Verification items for the finished model (mm, model axes). Coordinates: 2 decimals unless noted, no trailing zeros. Order: outer loops, then holes, each group sorted by start corner. A loop starts at its lowest first (then second) coordinate and runs counter-clockwise, first axis right, second up. Notation, with made-up numbers: M 27.5,-29.75 L 56.5,-29.75 A16 ccw 56.5,-21.75 Z; hole C 85,12.5 d6. An arc over 180 degrees is marked long. Return JSON: item names as keys, results as strings. Group by question number.
1. Material ranges on line 1 along X through (y, z) = (0.95, 76.2); line 2 along Z through (x, y) = (-88.9, 1); line 3 along Z through (x, y) = (9, 0.3), recorded low to high.
2. Section check A-A, the plane z = -36.5. Record the cut outline in (x, y).
3. Section check B-B, the plane x = -46.5. Record the cut outline in (y, z).
4. Gauge pin test, flat end, axial feed: pin 1 (1.8 mm diameter, centred on x = -88.9, z = 76.2, fed in from -Y). Record the tip position at first contact, or that the pin passes through.
5. Section check C-C, the plane y = 0.4. Give the number of separate pieces and of enclosed holes in the cut face, plus the area to 3 significant figures.
```python
from build123d import *

# Parameters (mm, degrees)
SKETCH1_W           = 203.2
SKETCH1_H           = 172.72
BOSS_EXTRUDE1_DEPTH = 1.5875
CUT_EXTRUDE1_DEPTH  = 1.5875
SKETCH3_R           = 1.5
CUT_EXTRUDE2_DEPTH  = 1.5875
FILLET1_R           = 10


with BuildPart() as part:
    # Sketch1 → Boss-Extrude1 (new body)
    with BuildSketch(Plane(origin=(0, 0, 0), x_dir=(1, 0, 0), z_dir=(0, 1, 0))):
        Rectangle(SKETCH1_W, SKETCH1_H)
    extrude(amount=BOSS_EXTRUDE1_DEPTH)

    # Sketch2 → Cut-Extrude1 (cut)
    with BuildSketch(Plane(origin=(0, 1.5875, 0), x_dir=(1, 0, 0), z_dir=(0, 1, 0))):
        with BuildLine():
            Line((-56.337811401, 60.96), (56.337811401, 60.96))
            ThreePointArc((56.337811401, 60.96), (61.186538483, 57.180592348), (58.70513907, 51.555938272))
            Line((58.70513907, 51.555938272), (14.203966015, 27.635097742))
            ThreePointArc((14.203966015, 27.635097742), (0, 24.059468112), (-14.203966015, 27.635097742))
            Line((-14.203966015, 27.635097742), (-58.70513907, 51.555938272))
            ThreePointArc((-58.70513907, 51.555938272), (-61.186538483, 57.180592348), (-56.337811401, 60.96))
        make_face()
        with BuildLine():
            Line((-56.337811401, -60.96), (56.337811401, -60.96))
            ThreePointArc((56.337811401, -60.96), (61.186538483, -57.180592348), (58.70513907, -51.555938272))
            Line((58.70513907, -51.555938272), (14.203966015, -27.635097742))
            ThreePointArc((14.203966015, -27.635097742), (0, -24.059468112), (-14.203966015, -27.635097742))
            Line((-14.203966015, -27.635097742), (-58.70513907, -51.555938272))
            ThreePointArc((-58.70513907, -51.555938272), (-61.186538483, -57.180592348), (-56.337811401, -60.96))
        make_face()
        with BuildLine():
            Line((-68.832672331, 20.873835416), (-41.470344365, 6.16568642))
            ThreePointArc((-41.470344365, 6.16568642), (-37.784603101, 0), (-41.470344365, -6.16568642))
            Line((-41.470344365, -6.16568642), (-68.832672331, -20.873835416))
            ThreePointArc((-68.832672331, -20.873835416), (-73.765478674, -20.761430614), (-76.2, -16.469773687))
            Line((-76.2, -16.469773687), (-76.2, 16.469773687))
            ThreePointArc((-76.2, 16.469773687), (-73.765478674, 20.761430614), (-68.832672331, 20.873835416))
        make_face()
        with BuildLine():
            Line((41.470344365, 6.16568642), (68.832672331, 20.873835416))
            ThreePointArc((68.832672331, 20.873835416), (73.765478674, 20.761430614), (76.2, 16.469773687))
            Line((76.2, 16.469773687), (76.2, -16.469773687))
            ThreePointArc((76.2, -16.469773687), (73.765478674, -20.761430614), (68.832672331, -20.873835416))
            Line((68.832672331, -20.873835416), (41.470344365, -6.16568642))
            ThreePointArc((41.470344365, -6.16568642), (37.784603101, 0), (41.470344365, 6.16568642))
        make_face()
    extrude(amount=-CUT_EXTRUDE1_DEPTH, mode=Mode.SUBTRACT)

    # Sketch3 → Cut-Extrude2 (cut)
    with BuildSketch(Plane(origin=(0, 1.5875, 0), x_dir=(1, 0, 0), z_dir=(0, 1, 0))):
        with Locations(Location((-88.9, 76.2, 0), (0, 0, 270))):
            Circle(SKETCH3_R)
        with Locations(Location((88.9, 76.2, 0), (0, 0, 270))):
            Circle(SKETCH3_R)
        with Locations(Location((88.9, -76.2, 0), (0, 0, 270))):
            Circle(SKETCH3_R)
        with Locations(Location((-88.9, -76.2, 0), (0, 0, 270))):
            Circle(SKETCH3_R)
    extrude(amount=-CUT_EXTRUDE2_DEPTH, mode=Mode.SUBTRACT)

    # Fillet1
    fillet1_edges = [part.edges().sort_by_distance(p)[0] for p in [
        (101.6, 0.79375, 86.36),
        (-101.6, 0.79375, 86.36),
        (-101.6, 0.79375, -86.36),
        (101.6, 0.79375, -86.36),
    ]]
    fillet(fillet1_edges, radius=FILLET1_R)


solid = part.part
```
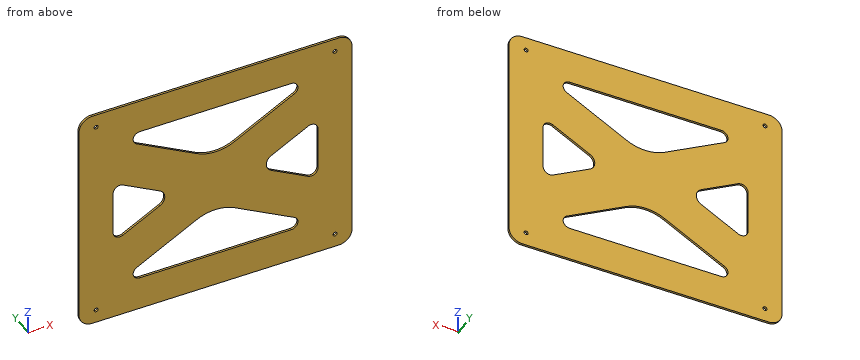
Answers follow:
{
 "1": {"line 1": "-101.6 to -90.4, -87.4 to 87.4, 90.4 to 101.6", "line 2": "-86.36 to -77.7, -74.7 to 74.7, 77.7 to 86.36", "line 3": "-86.36 to -60.96, -25.44 to 25.44, 60.96 to 86.36"},
 "2": {"outline": "M -101.6,0 L -30.7,0 L -30.7,1.59 L -101.6,1.59 Z; M 30.7,0 L 101.6,0 L 101.6,1.59 L 30.7,1.59 Z"},
 "3": {"outline": "M 0,-86.36 L 1.59,-86.36 L 1.59,-60.96 L 0,-60.96 Z; M 0,-45 L 1.59,-45 L 1.59,-8.87 L 0,-8.87 Z; M 0,8.87 L 1.59,8.87 L 1.59,45 L 0,45 Z; M 0,60.96 L 1.59,60.96 L 1.59,86.36 L 0,86.36 Z"},
 "4": {"pin 1": "through"},
 "5": {"separate pieces": "1", "enclosed holes": "8", "area": "26,900 mm^2"}
}
